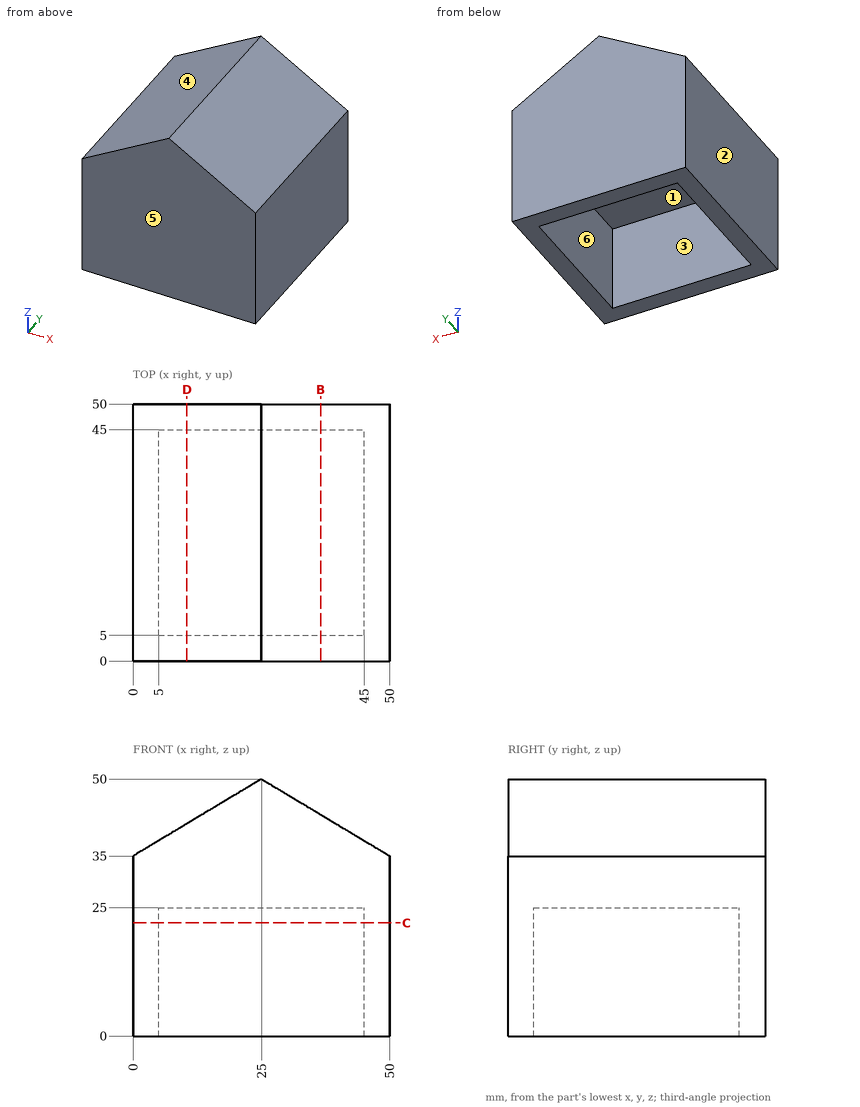
Job drawing, mm, ordinate dimensions from the low corner. One solid piece. A direction names the side the tool comes from. Round coordinates to 2 decimals unless told otherwise and drop trailing zeros. Loops run counter-clockwise (first coordinate to the right, second up) from the corner with the lowest first, then second, coordinate; pieces in that order, holes last.
(1) Two-plate mould, pull along X, no slides. Class the marked faces 3, 4, 5 and 6: +X half, -X half, draft (parallel to the pull), parting line (faces both ways), or undercut.
(2) Drop flat-ended pins along their axis: pin 1 (1.5 mm diameter, centred on y = 10, z = 44, fed in from -X); pin 2 (3 mm diameter, centred on x = 22.5, y = 7.5, fed in from +Z); pin 3 (3 mm diameter, centred on x = 11, y = 10.5, fed in from +Z); pin 4 (4 mm diameter, centred on y = 28.5, z = 6.5, fed in from -X). Give the stop position or say it passes through.
(3) Cut at C-C (z = 22). Give the cut face in (x, y), plus the area to 3 significant figures.
(4) Cut at D-D (x = 10.5). Give the cut face in (y, z).
(5) Cut at B-B (x = 36.5). Give the cut face in (y, z), plus the area to 4 significant figures.
(6) Which spindle directions (+Z, -Z, +X, -X, +Y, -Y) get a long thin tool onto all of the face, cutting with end or side? Do the marked faces 1 and 2. Say none if no direction does.
(7) Wall check: line 1 along X through (y, z) = (32, 12.5); line 2 along Z through (x, y) = (25, 38.5). Give the ranges that are in metal, low to high.
Findings below:
1. face 3: undercut
1. face 4: -X half
1. face 5: draft
1. face 6: undercut
2. pin 1: stops at x = 13.75
2. pin 2: stops at z = 49.4
2. pin 3: stops at z = 42.5
2. pin 4: stops at x = 0
3. outline: (0, 0) - (50, 0) - (50, 50) - (0, 50) - close; hole (5, 5) - (45, 5) - (45, 45) - (5, 45) - close
3. area: 900 mm2
4. outline: (0, 0) - (5, 0) - (5, 25) - (45, 25) - (45, 0) - (50, 0) - (50, 41.3) - (0, 41.3) - close
5. outline: (0, 0) - (5, 0) - (5, 25) - (45, 25) - (45, 0) - (50, 0) - (50, 43.1) - (0, 43.1) - close
5. area: 1,155 mm2
6. face 1: -Z
6. face 2: +Z, -Z, -X, +Y, -Y
7. line 1: x = 0 to 5, 45 to 50
7. line 2: z = 25 to 50
